Work out the finished part from the listing and answer in its coordinate system (mm). Coordinates: 2 decimals unless noted, no trailing zeros. Order: outer loops, then holes, each group sorted by start corner. A loop starts at its lowest first (then second) coordinate and runs counter-clockwise, first axis right, second up.
1. Determine the mould class of faces 1 (the flat face through (5, 1, 2)), 2 (the flat face through (-0.1, 0.4, -150)) for opening direction X: +X half, -X half, draft (parallel to the pull), parting line (faces both ways), or undercut.
2. Flat-ended cylindrical pins translate along their axes: pin 1 Ø2.5 at (x, z) = (-15, -10) entering from -Y; pin 2 Ø2 at (x, z) = (5, -61.5) entering from +Y; pin 3 Ø3 at (y, z) = (3, 71) entering from -X. Find the tip coordinate at first contact, or state that the pin passes through.
3. Find the intervals of material crossed by probe 1 along X at (y, z) = (5.25, 83); probe 2 along Y at (x, z) = (-8.5, 81); probe 3 along X at (y, z) = (1.5, -73), in increasing order.
4. The part is cut by section A-A, the plane z = -10. Give the vertices of the cut face in (x, y), then the cut area to 3 significant figures.
```python
from build123d import *

# Parameters (mm, degrees)
PAD_DEPTH           = 150
POCKET_DEPTH        = 5
LINEARPATTERN_COUNT = 11
LINEARPATTERN_PITCH = 27.5


with BuildPart() as part:
    # Sketch → Pad (new body, symmetric)
    with BuildSketch(Plane.XY):
        with BuildLine():
            Line((-11.7, 0), (11.7, 0))
            ThreePointArc((11.7, 0), (12.972792, 0.527208), (13.5, 1.8))
            Line((13.5, 1.8), (13.5, 5.7))
            ThreePointArc((14.3, 6.5), (13.734315, 6.265685), (13.5, 5.7))
            Line((14.3, 6.5), (17.5, 6.5))
            Line((17.5, 6.5), (17.5, 7.5))
            Line((17.5, 7.5), (14.3, 7.5))
            ThreePointArc((14.3, 7.5), (13.027208, 6.972792), (12.5, 5.7))
            Line((12.5, 5.7), (12.5, 1.8))
            ThreePointArc((11.7, 1), (12.265685, 1.234315), (12.5, 1.8))
            Line((11.7, 1), (-11.7, 1))
            ThreePointArc((-12.5, 1.8), (-12.265685, 1.234315), (-11.7, 1))
            Line((-12.5, 1.8), (-12.5, 5.7))
            ThreePointArc((-12.5, 5.7), (-13.027208, 6.972792), (-14.3, 7.5))
            Line((-14.3, 7.5), (-17.5, 7.5))
            Line((-17.5, 7.5), (-17.5, 6.5))
            Line((-17.5, 6.5), (-14.3, 6.5))
            ThreePointArc((-13.5, 5.7), (-13.734315, 6.265685), (-14.3, 6.5))
            Line((-13.5, 5.7), (-13.5, 1.8))
            ThreePointArc((-13.5, 1.8), (-12.972792, 0.527208), (-11.7, 0))
        make_face()
    extrude(amount=PAD_DEPTH, both=True)

    # Sketch001 (on Face13 of Pad) → Pocket (cut)
    with BuildSketch(Plane(origin=(0, 1, 0), x_dir=(-1, 0, 0), z_dir=(0, 1, 0))):
        with BuildLine():
            ThreePointArc((-2.9, -140), (0, -142.9), (2.9, -140))
            Line((2.9, -140), (2.9, -126))
            ThreePointArc((2.9, -126), (0, -123.1), (-2.9, -126))
            Line((-2.9, -140), (-2.9, -126))
        make_face()
    pocket = extrude(amount=-POCKET_DEPTH, mode=Mode.SUBTRACT)

    # LinearPattern: Pocket ×11
    with Locations(*[(0, 0, i * LINEARPATTERN_PITCH) for i in range(1, LINEARPATTERN_COUNT)]):
        add(pocket, mode=Mode.SUBTRACT)


solid = part.part
```
Geometry says:
1. face 1: undercut
1. face 2: draft
2. pin 1: stops at y = 6.28
2. pin 2: stops at y = 1
2. pin 3: stops at x = -13.5
3. probe 1: x = -13.5 to -12.5, 12.5 to 13.5
3. probe 2: y = 0 to 1
3. probe 3: x = -13.47 to -12.44, 12.44 to 13.47
4. outline: (-17.5, 6.5) - (-14.3, 6.5) arc R0.8 cw to (-13.5, 5.7) - (-13.5, 1.8) arc R1.8 ccw to (-11.7, 0) - (11.7, 0) arc R1.8 ccw to (13.5, 1.8) - (13.5, 5.7) arc R0.8 cw to (14.3, 6.5) - (17.5, 6.5) - (17.5, 7.5) - (14.3, 7.5) arc R1.8 ccw to (12.5, 5.7) - (12.5, 1.8) arc R0.8 cw to (11.7, 1) - (-11.7, 1) arc R0.8 cw to (-12.5, 1.8) - (-12.5, 5.7) arc R1.8 ccw to (-14.3, 7.5) - (-17.5, 7.5) - close
4. area: 45.8 mm2
